Geometry check sheet. Reference: the model listing, model coordinates, mm. Face numbers are marked on the shaded views. Round coordinates to 2 decimals unless told otherwise and drop trailing zeros. Order: outer loops, then holes, each group sorted by start corner. A loop starts at its lowest first (then second) coordinate and runs counter-clockwise, first axis right, second up. Notation, with made-up numbers: (5, 58.5) - (59, 58.5) arc R20 ccw to (59, 73.5) - close; hole circle Ø1 at (-36, 57.5). An arc over 180 degrees is marked (long way). Use a Markdown table: item, result. Add a question column.
(1) Section check C-C on x = 8.25. Record the boundary of the cut face in (y, z), then the cut area to 3 significant figures.
(2) Mould release check, pull along Y, two halves, no side actions. Record for the marked faces 1, 2 and 3: released by +Y, released by -Y, zero draft, split by the parting line, or undercut.
(3) Section check A-A on z = 0. Record the boundary of the cut face in (x, y).
(4) Gauge pin test, flat ends, axial feed: P1, Ø5, axis at x = 8, y = 4, coming from the -Z side; P2, Ø3, axis at x = 5.5, y = -7, coming from the -Z side; P3, Ø1, axis at x = 7.5, y = -7.5, coming from the -Z side. Record the tip position at first contact, or that the pin passes through.
(5) Thickness scan on line 1 along Z through (x, y) = (2, 0); line 2 along Y through (x, z) = (3, 3); line 3 along Y through (x, z) = (1, -3.5). Record the ranges inside material, lowest first. Write a range as [from, to].
Autodesk Inventor part; units mm, degrees
ref_plane "YZ Plane" through (0, 0, 0) normal (1, 0, 0) x (0, 1, 0)
ref_plane "XZ Plane" through (0, 0, 0) normal (0, 1, 0) x (-1, 0, 0)
ref_plane "XY Plane" through (0, 0, 0) normal (0, 0, 1) x (1, 0, 0)
sketch "Sketch_1" plane through (0, 0, 0) normal (0, 0, 1) x (1, 0, 0)
  line L0 (50, 0) -> (-50, 0)
  arc A0 (0, 7.8) -> (0.3, 7.5) centre (0.3, 7.8) ccw
  line L1 (0.3, 7.5) -> (8.7, 7.5)
  arc A1 (8.7, 7.5) -> (9, 7.8) centre (8.7, 7.8) ccw
  line L2 (9, 7.8) -> (9, 10.25)
  line L3 (9, 10.25) -> (6.3491, 10.25)
  arc A2 (2.6509, 10.25) -> (6.3491, 10.25) centre (4.5, 11.75) ccw
  line L4 (2.6509, 10.25) -> (0, 10.25)
  line L5 (0, 10.25) -> (0, 7.8)
revolve "Revolution1" add sketch "Sketch_1" angle 360 about axis through (50, 0, 0) along (1, 0, 0)
properties part number "6002_PART1"
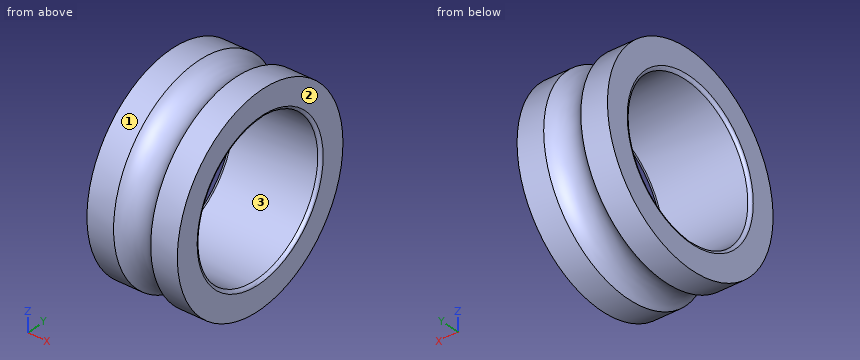
Check sheet entries:
| question | item | result |
|---|---|---|
| 1 | outline | circle Ø20.5 at (0, 0); hole circle Ø15 at (0, 0) |
| 1 | area | 153 mm2 |
| 2 | face 1 | split by the parting line |
| 2 | face 2 | zero draft |
| 2 | face 3 | undercut |
| 3 | outline | (0, -10.25) - (2.65, -10.25) arc R2.38 cw to (6.35, -10.25) - (9, -10.25) - (9, -7.8) arc R0.3 ccw to (8.7, -7.5) - (0.3, -7.5) arc R0.3 ccw to (0, -7.8) - close; (0, 7.8) arc R0.3 ccw to (0.3, 7.5) - (8.7, 7.5) arc R0.3 ccw to (9, 7.8) - (9, 10.25) - (6.35, 10.25) arc R2.38 cw to (2.65, 10.25) - (0, 10.25) - close |
| 4 | P1 | stops at z = -10.14 |
| 4 | P2 | stops at z = -8.48 |
| 4 | P3 | stops at z = -7.49 |
| 5 | line 1 | z = [-10.25, -7.5], [7.5, 10.25] |
| 5 | line 2 | y = [-9.44, -6.87], [6.87, 9.44] |
| 5 | line 3 | y = [-9.63, -6.63], [6.63, 9.63] |
